Print and shaded views of the part. All mm, measured from the part's lowest x, y and z. A direction names the side the tool comes from. Round coordinates to 2 decimals unless told otherwise and drop trailing zeros. Order: outer loops, then holes, each group sorted by start corner. A loop starts at its lowest first (then second) coordinate and runs counter-clockwise, first axis right, second up. Notation, with made-up numbers: (52, 83.25) - (64, 83.25) arc R16 cw to (64, 93.25) - close; hole circle Ø7 at (62.25, -9). An arc over 180 degrees is marked (long way). Return JSON: item names as keys, results as strings. Group by question number.
Item 1: Saw through at C-C on y = 17.5. List the corners of the cut face in (x, z) (3 decimals).
Item 2: Two-plate mould, pull along X, no slides. Class the marked faces 1, 2 and 3: released by +X, released by -X, zero draft, split by the parting line, or undercut.
Item 3: Saw through at B-B on z = 38.1. List the corners of the cut face in (x, y) (3 decimals), and give its area (3 significant figures).
Item 4: Probe probe 1 along Z at (x, y) = (38.1, 27.75) (3 decimals); probe 2 along X at (y, z) = (20, 38); probe 3 along Z at (x, y) = (38.1, 2.5). List the from-to ranges inside material, lowest first.
Item 5: Saw through at A-A on x = 38.1. List the corners of the cut face in (y, z) (3 decimals), and give its area (3 significant figures).
Item 6: Tool access for the marked faces 4 and 5: list every direction of +Z, -Z, +X, -X, +Y, -Y with a clear straight run to the whole face (end or side of a thin tool).
Item 7: Drop flat-ended pins along their axis: pin 1 (10 mm diameter, centred on x = 26, y = 10, fed in from -Z); pin 2 (4 mm diameter, centred on y = 7.5, z = 25.5, fed in from -X); pin 3 (8.5 mm diameter, centred on x = 57.15, z = 38.1, fed in from -Y). Give the stop position or say it passes through.
Item 8: Saw through at D-D on z = 19.05. List the corners of the cut face in (x, y) (3 decimals), and give its area (3 significant figures).
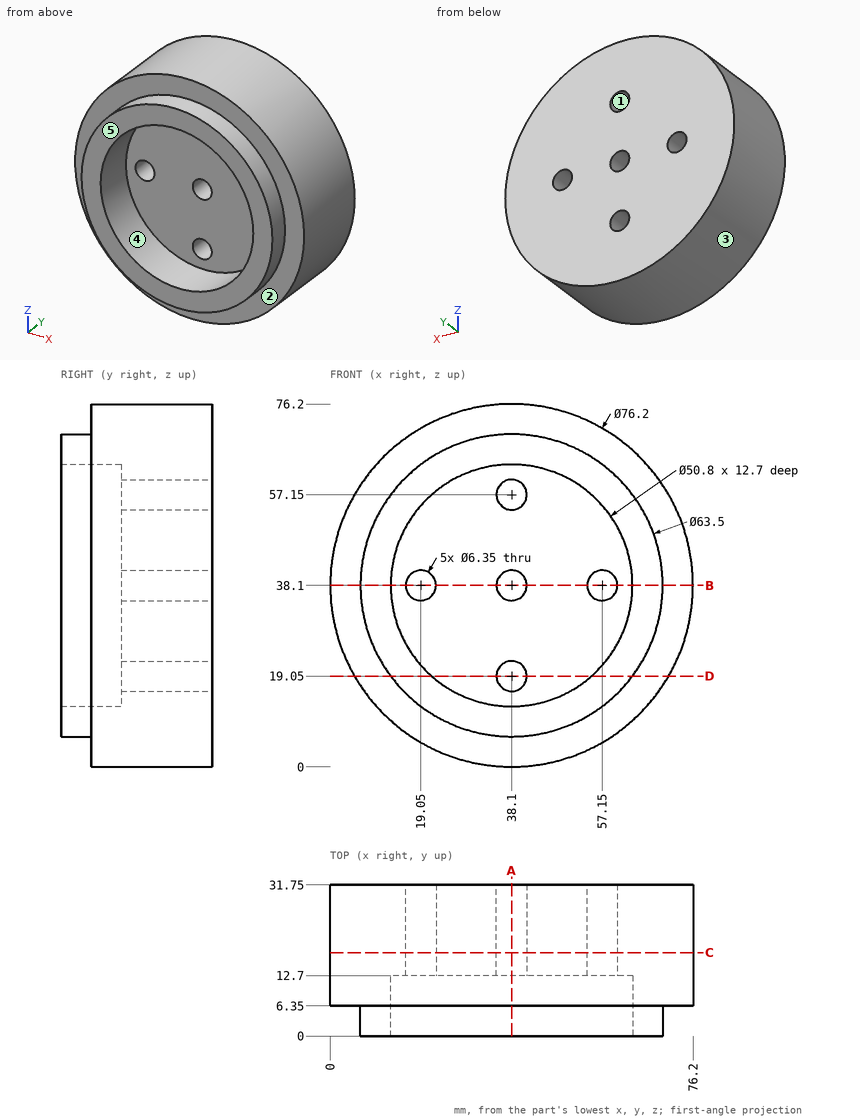
Filled in:
{
 "1": {"outline": "circle Ø76.2 at (38.1, 38.1); hole circle Ø6.35 at (19.05, 38.1); hole circle Ø6.35 at (38.1, 19.05); hole circle Ø6.35 at (38.1, 38.1); hole circle Ø6.35 at (38.1, 57.15); hole circle Ø6.35 at (57.15, 38.1)"},
 "2": {"face 1": "undercut", "face 2": "zero draft", "face 3": "split by the parting line"},
 "3": {"outline": "(0, 6.35) - (6.35, 6.35) - (6.35, 0) - (12.7, 0) - (12.7, 12.7) - (15.875, 12.7) - (15.875, 31.75) - (0, 31.75) - close; (22.225, 12.7) - (34.925, 12.7) - (34.925, 31.75) - (22.225, 31.75) - close; (41.275, 12.7) - (53.975, 12.7) - (53.975, 31.75) - (41.275, 31.75) - close; (60.325, 12.7) - (63.5, 12.7) - (63.5, 0) - (69.85, 0) - (69.85, 6.35) - (76.2, 6.35) - (76.2, 31.75) - (60.325, 31.75) - close", "area": "1,330 mm^2"},
 "4": {"probe 1": "z = 0 to 15.875, 22.225 to 34.925, 41.275 to 53.975, 60.325 to 76.2", "probe 2": "x = 0 to 15.88, 22.22 to 34.93, 41.27 to 53.98, 60.32 to 76.2", "probe 3": "z = 6.35 to 12.7, 63.5 to 69.85"},
 "5": {"outline": "(0, 6.35) - (6.35, 6.35) - (6.35, 0) - (31.75, 0) - (31.75, 15.875) - (12.7, 15.875) - (12.7, 12.7) - (0, 12.7) - close; (0, 63.5) - (12.7, 63.5) - (12.7, 60.325) - (31.75, 60.325) - (31.75, 76.2) - (6.35, 76.2) - (6.35, 69.85) - (0, 69.85) - close; (12.7, 22.225) - (31.75, 22.225) - (31.75, 34.925) - (12.7, 34.925) - close; (12.7, 41.275) - (31.75, 41.275) - (31.75, 53.975) - (12.7, 53.975) - close", "area": "1,330 mm^2"},
 "6": {"face 4": "-Y", "face 5": "+Z, -Z, +X, -X, -Y"},
 "7": {"pin 1": "stops at z = 0.67", "pin 2": "stops at x = 1.5", "pin 3": "stops at y = 12.7"},
 "8": {"outline": "(5.104, 6.35) - (12.7, 6.35) - (12.7, 0) - (21.299, 0) - (21.299, 12.7) - (34.925, 12.7) - (34.925, 31.75) - (5.104, 31.75) - close; (41.275, 12.7) - (54.901, 12.7) - (54.901, 0) - (63.5, 0) - (63.5, 6.35) - (71.096, 6.35) - (71.096, 31.75) - (41.275, 31.75) - close", "area": "1,450 mm^2"}
}
